```python
from build123d import *

# Parameters (mm, degrees)
BOSS_EXTRUDE1_DEPTH = 6
SKETCH3_W           = 19
SKETCH3_H           = 6
SKETCH3_W_2         = 6
SKETCH3_H_2         = 19
CUT_EXTRUDE1_DEPTH  = 71.964779997
SKETCH4_W           = 6
SKETCH4_H           = 6
CUT_EXTRUDE2_DEPTH  = 71.964779997


with BuildPart() as part:
    # Sketch2 → Boss-Extrude1 (new body)
    with BuildSketch(Plane(origin=(0, 0, 0), x_dir=(1, 0, 0), z_dir=(0, 1, 0))):
        Polygon((0, 0), (-10, 0), (-10, 12), (-50, 12), (12, -50), (12, -10), (0, -10), align=None)
    extrude(amount=BOSS_EXTRUDE1_DEPTH)

    # Sketch3 → Cut-Extrude1 (cut, through all)
    with BuildSketch(Plane(origin=(0, 6, 0), x_dir=(1, 0, 0), z_dir=(0, 1, 0))):
        with Locations((-34.5, 3)):
            Rectangle(SKETCH3_W, SKETCH3_H)
        with Locations((3, -34.5)):
            Rectangle(SKETCH3_W_2, SKETCH3_H_2)
    extrude(amount=-CUT_EXTRUDE1_DEPTH, mode=Mode.SUBTRACT)

    # Sketch4 → Cut-Extrude2 (cut, through all)
    with BuildSketch(Plane(origin=(0, 6, 0), x_dir=(1, 0, 0), z_dir=(0, 1, 0))):
        with Locations((-47, 9)):
            Rectangle(SKETCH4_W, SKETCH4_H)
        with Locations((9, -47)):
            Rectangle(SKETCH4_W, SKETCH4_H)
    extrude(amount=-CUT_EXTRUDE2_DEPTH, mode=Mode.SUBTRACT)


solid = part.part
```
CAD build for the part. Positions are in the model's coordinates, mm. A direction names the side the tool comes from. Give positions to 0.01 mm unless a question says otherwise; leave off trailing zeros. Order: outer loops, then holes, each group sorted by start corner. A loop starts at its lowest first (then second) coordinate and runs counter-clockwise, first axis right, second up.
(1) Saw through at C-C, the plane y = 1.55. Give the cut face in (x, z).
(2) Drill centre lines: L1, parallel to X at y = 3.9, z = 38.5; L2, parallel to X at y = 5.45, z = 33; L3, parallel to Z at x = -40, y = 1.55. Where is each one in solid material? Low to high.
(3) Saw through at A-A, the plane x = -33. Give the cut face in (y, z), then the cut area to 3 significant figures.
(4) Tool access for faces 1 (the flat face through (3, 3, 25)), 2 (the flat face through (0, 3, 5)), 3 (the flat face through (-44, 3, -9)), 4 (the flat face through (-35, 3, -6)): list every direction of +Z, -Z, +X, -X, +Y, -Y with a clear straight run to the whole face (end or side of a thin tool).
(5) Mould opens along Z. For faces 5 (the flat face through (-25, 3, -3)), 6 (the flat face through (6, 3, 10)), 7 (the flat face through (0, 3, 32)) say: released by +Z, released by -Z, zero draft, split by the parting line, or undercut.
(6) Flat gauge pins, fed straight in: pin 1 (3 mm diameter, centred on y = 3, z = 30.5, fed in from -X); pin 2 (1.8 mm diameter, centred on x = -37, y = 3.5, fed in from +Z); pin 3 (1.8 mm diameter, centred on y = 2.5, z = 3.5, fed in from +X); pin 4 (5 mm diameter, centred on x = -27.5, z = 17.5, fed in from -Y). Where does each tip first touch, or does it go through?
(7) Saw through at D-D, the plane x = 2.5. Give the cut face in (y, z), then the cut area to 3 significant figures.
(8) Saw through at B-B, the plane z = 27.5. Give the cut face in (x, y), then the cut area to 3 significant figures.
Results found:
1. outline: (-44, -12) - (-10, -12) - (-10, 0) - (0, 0) - (0, 10) - (12, 10) - (12, 44) - (6, 44) - (6, 25) - (0, 25) - (0, 38) - (-38, 0) - (-25, 0) - (-25, -6) - (-44, -6) - close
2. L1: x = 6 to 12
2. L2: x = -5 to 0, 6 to 12
2. L3: z = -12 to -6
3. outline: (0, -12) - (6, -12) - (6, -6) - (0, -6) - close; (0, 0) - (6, 0) - (6, 5) - (0, 5) - close
3. area: 66.0 mm2
4. face 1: +Z, +Y, -Y
4. face 2: -Z, +X, +Y, -Y
4. face 3: +Z, -Z, -X, +Y, -Y
4. face 4: -X, +Y, -Y
5. face 5: undercut
5. face 6: released by -Z
5. face 7: zero draft
6. pin 1: stops at x = -9
6. pin 2: stops at z = 1.9
6. pin 3: stops at x = 0
6. pin 4: passes through
7. outline: (0, 10) - (6, 10) - (6, 25) - (0, 25) - close
7. area: 90.0 mm2
8. outline: (-10.5, 0) - (0, 0) - (0, 6) - (-10.5, 6) - close; (6, 0) - (12, 0) - (12, 6) - (6, 6) - close
8. area: 99.0 mm2
